CAD build for the part. Positions are in the model's coordinates, mm. A direction names the side the tool comes from. Coordinates: 2 decimals unless noted, no trailing zeros. Write each loop counter-clockwise with the first axis right and the second up, starting at its lowest first coordinate (ties: lowest second). Pieces come first, ordered by that corner, then holes. Notation, with made-up numbers: (22.25, -26) - (29.25, -26) arc R28 ccw to (29.25, 4) - close; hole circle Ø11 at (51.25, 54). An arc over 180 degrees is marked (long way). One line per question, with ' | ' between items. Start each with the question number.
1. Band-saw the part on C-C, the plane x = 12.5. Write the cut outline in (y, z), then the cut area to 3 significant figures.
2. Two-plate mould, pull along X, no slides. Class faces 1 (the cylindrical face through (49.56, 111.044, 7.549)), 2 (the flat face through (76.2, 63, 1)), 3 (the flat face through (40, 18, -12.7)), 4 (the flat face through (0, 48, 4)): +X half, -X half, draft (parallel to the pull), parting line (faces both ways), or undercut.
3. Probe line 1 (Y direction, x = 50.8, z = 6.5) (3 decimals); line 2 (X direction, y = 48.5, z = 6.5). List the from-to ranges inside material, lowest first.
4. Band-saw the part on B-B, the plane x = 50.8. Write the cut outline in (y, z) (3 decimals).
5. Band-saw the part on D-D, the plane y = 29. Write the cut outline in (x, z), then the cut area to 3 significant figures.
6. Flat gauge pins, fed straight in: P1, Ø11, axis at x = 43, z = -6, coming from the +Y side; P2, Ø4, axis at x = 42, y = 14, coming from the +Z side; P3, Ø3, axis at y = 25, z = -0.5, coming from the +X side; P4, Ø11.5, axis at x = 50.8, y = 101.6, coming from the -Z side. Where does each tip first touch, or does it go through?
7. Band-saw the part on A-A, the plane z = 6. Write the cut outline in (x, y) (3 decimals), then the cut area to 3 significant figures.
8. Which spindle directions (+Z, -Z, +X, -X, +Y, -Y) get a long thin tool onto all of the face, cutting with end or side? Do faces 5 (the flat face through (39, 35.56, -4)), 6 (the flat face through (39, 82, 0)), 7 (the flat face through (60, 105, 12.7)). Say none if no direction does.
from build123d import *

# Parameters (mm, degrees)
SKETCH1_W           = 76.2
SKETCH1_H           = 127
BOSS_EXTRUDE2_DEPTH = 12.7
SKETCH2_W           = 76.2
SKETCH2_H           = 38.1
BOSS_EXTRUDE3_DEPTH = 12.7
SKETCH4_R           = 9.525
CUT_EXTRUDE1_DEPTH  = 149.649688866
FILLET1_R           = 2.54
CHAMFER1_SIZE       = 2.54
SHELL1_START        = 2.54
SHELL1_DEPTH        = 73.66
SHELL1_START_2      = 35.56
SHELL1_3_DEPTH      = 89.44
SHELL1_4_DEPTH      = 35.56


with BuildPart() as part:
    # Sketch1 → Boss-Extrude2 (new body)
    with BuildSketch(Plane.XY):
        with Locations((38.1, 63.5)):
            Rectangle(SKETCH1_W, SKETCH1_H)
    extrude(amount=BOSS_EXTRUDE2_DEPTH)

    # Sketch2 → Boss-Extrude3 (add)
    with BuildSketch(Plane(origin=(0, 0, 0), x_dir=(-1, 0, 0), z_dir=(0, 0, -1))):
        with Locations((-38.1, 19.05)):
            Rectangle(SKETCH2_W, SKETCH2_H)
    extrude(amount=BOSS_EXTRUDE3_DEPTH)

    # Sketch4 → Cut-Extrude1 (cut, through all)
    with BuildSketch(Plane(origin=(0, 0, 0), x_dir=(-1, 0, 0), z_dir=(0, 0, -1))):
        with Locations((-50.8, 101.6)):
            Circle(SKETCH4_R)
    extrude(amount=-CUT_EXTRUDE1_DEPTH, mode=Mode.SUBTRACT)

    # Fillet1
    fillet1_edges = [part.edges().sort_by_distance(p)[0] for p in [
        (0, 38.1, -6.35),
        (0, 127, 6.35),
    ]]
    fillet(fillet1_edges, radius=FILLET1_R)

    # Chamfer1
    chamfer1_edges = [part.edges().sort_by_distance(p)[0] for p in [
        (60.325, 101.6, 0),
        (0, 80.01, 0),
        (0.743948776, 126.256051224, 0),
        (39.37, 127, 0),
        (0, 17.78, -12.7),
        (0.743948776, 37.356051224, -12.7),
        (39.37, 38.1, -12.7),
    ]]
    chamfer(chamfer1_edges, length=CHAMFER1_SIZE)

    # Shell1: read off the stored shape, not the designer's step
    # Shell1 outline → Shell1 (cut)
    with BuildSketch(Plane.YZ.offset(SHELL1_START)):
        Polygon((124.46, 3.592102448), (124.46, 12.7), (0, 12.7), (0, -10.16), (34.507897552, -10.16), (35.56, -9.107897552), (35.56, 2.54), (123.407897552, 2.54), align=None)
    extrude(amount=SHELL1_DEPTH, mode=Mode.SUBTRACT)

    # Shell1 2 outline → Shell1 2 (revolve)
    with BuildSketch(Plane(origin=(50.8, 101.6, 0), x_dir=(1, 0, 0), z_dir=(0, -1, 0))):
        Polygon((12.065, 12.7), (9.525, 12.7), (9.525, 2.54), (13.117102448, 2.54), (12.065, 3.592102448), align=None)
    revolve(axis=Axis((50.8, 101.6, 0), (0, 0, 1)))

    # Shell1 3 outline → Shell1 3 (add)
    with BuildSketch(Plane(origin=(0, 0, 0), x_dir=(1, 0, 0), z_dir=(0, 1, 0)).offset(SHELL1_START_2)):
        Polygon((2.54, -3.592102448), (3.592102448, -2.54), (2.54, -2.54), align=None)
    extrude(amount=SHELL1_3_DEPTH)

    # Shell1 4 outline → Shell1 4 (add)
    with BuildSketch(Plane(origin=(0, 0, 0), x_dir=(1, 0, 0), z_dir=(0, 1, 0))):
        Polygon((2.54, 10.16), (2.54, 9.107897552), (3.592102448, 10.16), align=None)
    extrude(amount=SHELL1_4_DEPTH)


solid = part.part
Filled in:
1) outline: (0, -12.7) - (35.56, -12.7) - (38.1, -10.16) - (38.1, 0) - (124.46, 0) - (127, 2.54) - (127, 12.7) - (124.46, 12.7) - (124.46, 3.59) - (123.41, 2.54) - (35.56, 2.54) - (35.56, -9.11) - (34.51, -10.16) - (0, -10.16) - close | area: 375 mm²
2) face 1: undercut | face 2: +X half | face 3: draft | face 4: -X half
3) line 1: y = 89.535 to 92.075, 111.125 to 113.665, 124.46 to 127 | line 2: x = 0 to 2.54
4) outline: (0, -12.7) - (35.56, -12.7) - (38.1, -10.16) - (38.1, 0) - (89.535, 0) - (92.075, 2.54) - (92.075, 12.7) - (89.535, 12.7) - (89.535, 3.592) - (88.483, 2.54) - (35.56, 2.54) - (35.56, -9.108) - (34.508, -10.16) - (0, -10.16) - close; (111.125, 2.54) - (113.665, 0) - (124.46, 0) - (127, 2.54) - (127, 12.7) - (124.46, 12.7) - (124.46, 3.592) - (123.408, 2.54) - (114.717, 2.54) - (113.665, 3.592) - (113.665, 12.7) - (111.125, 12.7) - close
5) outline: (0, -10.16) - (2.54, -12.7) - (76.2, -12.7) - (76.2, -10.16) - (3.59, -10.16) - (2.54, -9.11) - (2.54, 12.7) - (0, 12.7) - close | area: 249 mm²
6) P1: stops at y = 38.1 | P2: stops at z = -10.16 | P3: stops at x = 2.54 | P4: passes through
7) outline: (0, 0) - (2.54, 0) - (2.54, 124.46) - (76.2, 124.46) - (76.2, 127) - (2.54, 127) arc R2.54 ccw to (0, 124.46) - close; circle Ø24.13 at (50.8, 101.6); hole circle Ø19.05 at (50.8, 101.6) | area: 681 mm²
8) face 5: +Z, +X, -Y | face 6: -Z, +X, -X, +Y | face 7: +Z, +X, -X, +Y, -Y
